For this review, take the finished solid that the model builds, in its own axes (mm). A direction names the side the tool comes from. Coordinates: 2 decimals unless noted, no trailing zeros. Write each loop counter-clockwise with the first axis right and the second up, starting at its lowest first coordinate (ties: lowest second). Pieces come first, ordered by that corner, then holes. Notation, with made-up numbers: M 53,13 L 79,13 A35 cw 79,48 Z; hole C 73.25,81.25 d11. An arc over 180 degrees is marked long. Return JSON: item names as keys, results as strings.
```python
from build123d import *

# Parameters (mm, degrees)
ESBO_O1_W                      = 4
ESBO_O1_H                      = 4
RESSALTO_EXTRUS_O1_DEPTH       = 100
PADR_OCIRCULAR1_COUNT          = 4
PADR_O_LINEAR1_COUNT           = 2
PADR_O_LINEAR1_PITCH           = 30
PADR_O_LINEAR1_COPY_1_SKETCH_W = 4
PADR_O_LINEAR1_COPY_1_SKETCH_H = 4
PADR_O_LINEAR1_COPY_1_DEPTH    = 100
PADR_O_LINEAR1_COPY_2_SKETCH_W = 4
PADR_O_LINEAR1_COPY_2_SKETCH_H = 4
PADR_O_LINEAR1_COPY_2_DEPTH    = 100
PADR_O_LINEAR1_COPY_3_SKETCH_W = 4
PADR_O_LINEAR1_COPY_3_SKETCH_H = 4
PADR_O_LINEAR1_COPY_3_DEPTH    = 100
ESBO_O4_W                      = 10
ESBO_O4_H                      = 28
CORTE_EXTRUS_O1_DEPTH          = 111.679718106
FILETE1_R                      = 1
CUT_EXTRUDE1_DEPTH             = 118.579760163


with BuildPart() as part:
    # Esboço1 → Ressalto-extrusão1 (new body)
    with BuildSketch(Plane.XY):
        with BuildLine():
            ThreePointArc((-1.664601464, 3.078815026), (-0.858529967, 3.393070335), (0, 3.5))
            Line((0, 3.5), (0, 6))
            Line((0, 6), (-3.878679656, 6))
            Line((-3.878679656, 6), (-8.5, 10.621320344))
            Line((-8.5, 10.621320344), (-8.5, 13))
            Line((-8.5, 13), (-4.1, 13))
            Line((-4.1, 13), (-4.1, 14.5))
            Line((-4.1, 14.5), (-5.1, 14.5))
            Line((-5.1, 14.5), (-5.1, 15))
            Line((-5.1, 15), (-15, 15))
            Line((-15, 15), (-15, 5.1))
            Line((-15, 5.1), (-14.5, 5.1))
            Line((-14.5, 5.1), (-14.5, 4.1))
            Line((-14.5, 4.1), (-13, 4.1))
            Line((-13, 4.1), (-13, 8.5))
            Line((-13, 8.5), (-10.621320344, 8.5))
            Line((-10.621320344, 8.5), (-6, 3.878679656))
            Line((-6, 3.878679656), (-6, 0))
            Line((-6, 0), (-3.5, 0))
            ThreePointArc((-3.5, 0), (-3.393070335, 0.858529967), (-3.078815026, 1.664601464))
            Line((-3.078815026, 1.664601464), (-4.596194078, 3.181980515))
            Line((-4.596194078, 3.181980515), (-3.181980515, 4.596194078))
            Line((-3.181980515, 4.596194078), (-1.664601464, 3.078815026))
        make_face()
        with Locations((-12, 12)):
            Rectangle(ESBO_O1_W, ESBO_O1_H, mode=Mode.SUBTRACT)
    ressalto_extrus_o1 = extrude(amount=RESSALTO_EXTRUS_O1_DEPTH)

    # PadrãoCircular1: Ressalto-extrusão1 ×4 about axis
    padr_ocircular1_axis = Axis((0, 0, 0), (0, 0, 1))
    for i in range(1, PADR_OCIRCULAR1_COUNT):
        add(ressalto_extrus_o1.rotate(padr_ocircular1_axis, i * 360 / PADR_OCIRCULAR1_COUNT))

    # Padrão linear1: Ressalto-extrusão1 ×2
    with Locations(*[(i * PADR_O_LINEAR1_PITCH, 0, 0) for i in range(1, PADR_O_LINEAR1_COUNT)]):
        add(ressalto_extrus_o1)

    # Padrão linear1 copy 1 sketch → Padrão linear1 copy 1 (add)
    with BuildSketch(Plane(origin=(30, 0, 0), x_dir=(0, 1, 0), z_dir=(0, 0, 1))):
        with BuildLine():
            ThreePointArc((-1.664601464, 3.078815026), (-0.858529967, 3.393070335), (0, 3.5))
            Line((0, 3.5), (0, 6))
            Line((0, 6), (-3.878679656, 6))
            Line((-3.878679656, 6), (-8.5, 10.621320344))
            Line((-8.5, 10.621320344), (-8.5, 13))
            Line((-8.5, 13), (-4.1, 13))
            Line((-4.1, 13), (-4.1, 14.5))
            Line((-4.1, 14.5), (-5.1, 14.5))
            Line((-5.1, 14.5), (-5.1, 15))
            Line((-5.1, 15), (-15, 15))
            Line((-15, 15), (-15, 5.1))
            Line((-15, 5.1), (-14.5, 5.1))
            Line((-14.5, 5.1), (-14.5, 4.1))
            Line((-14.5, 4.1), (-13, 4.1))
            Line((-13, 4.1), (-13, 8.5))
            Line((-13, 8.5), (-10.621320344, 8.5))
            Line((-10.621320344, 8.5), (-6, 3.878679656))
            Line((-6, 3.878679656), (-6, 0))
            Line((-6, 0), (-3.5, 0))
            ThreePointArc((-3.5, 0), (-3.393070335, 0.858529967), (-3.078815026, 1.664601464))
            Line((-3.078815026, 1.664601464), (-4.596194078, 3.181980515))
            Line((-4.596194078, 3.181980515), (-3.181980515, 4.596194078))
            Line((-3.181980515, 4.596194078), (-1.664601464, 3.078815026))
        make_face()
        with Locations((-12, 12)):
            Rectangle(PADR_O_LINEAR1_COPY_1_SKETCH_W, PADR_O_LINEAR1_COPY_1_SKETCH_H, mode=Mode.SUBTRACT)
    extrude(amount=PADR_O_LINEAR1_COPY_1_DEPTH)

    # Padrão linear1 copy 2 sketch → Padrão linear1 copy 2 (add)
    with BuildSketch(Plane(origin=(30, 0, 0), x_dir=(-1, 0, 0), z_dir=(0, 0, 1))):
        with BuildLine():
            ThreePointArc((-1.664601464, 3.078815026), (-0.858529967, 3.393070335), (0, 3.5))
            Line((0, 3.5), (0, 6))
            Line((0, 6), (-3.878679656, 6))
            Line((-3.878679656, 6), (-8.5, 10.621320344))
            Line((-8.5, 10.621320344), (-8.5, 13))
            Line((-8.5, 13), (-4.1, 13))
            Line((-4.1, 13), (-4.1, 14.5))
            Line((-4.1, 14.5), (-5.1, 14.5))
            Line((-5.1, 14.5), (-5.1, 15))
            Line((-5.1, 15), (-15, 15))
            Line((-15, 15), (-15, 5.1))
            Line((-15, 5.1), (-14.5, 5.1))
            Line((-14.5, 5.1), (-14.5, 4.1))
            Line((-14.5, 4.1), (-13, 4.1))
            Line((-13, 4.1), (-13, 8.5))
            Line((-13, 8.5), (-10.621320344, 8.5))
            Line((-10.621320344, 8.5), (-6, 3.878679656))
            Line((-6, 3.878679656), (-6, 0))
            Line((-6, 0), (-3.5, 0))
            ThreePointArc((-3.5, 0), (-3.393070335, 0.858529967), (-3.078815026, 1.664601464))
            Line((-3.078815026, 1.664601464), (-4.596194078, 3.181980515))
            Line((-4.596194078, 3.181980515), (-3.181980515, 4.596194078))
            Line((-3.181980515, 4.596194078), (-1.664601464, 3.078815026))
        make_face()
        with Locations((-12, 12)):
            Rectangle(PADR_O_LINEAR1_COPY_2_SKETCH_W, PADR_O_LINEAR1_COPY_2_SKETCH_H, mode=Mode.SUBTRACT)
    extrude(amount=PADR_O_LINEAR1_COPY_2_DEPTH)

    # Padrão linear1 copy 3 sketch → Padrão linear1 copy 3 (add)
    with BuildSketch(Plane(origin=(30, 0, 0), x_dir=(0, -1, 0), z_dir=(0, 0, 1))):
        with BuildLine():
            ThreePointArc((-1.664601464, 3.078815026), (-0.858529967, 3.393070335), (0, 3.5))
            Line((0, 3.5), (0, 6))
            Line((0, 6), (-3.878679656, 6))
            Line((-3.878679656, 6), (-8.5, 10.621320344))
            Line((-8.5, 10.621320344), (-8.5, 13))
            Line((-8.5, 13), (-4.1, 13))
            Line((-4.1, 13), (-4.1, 14.5))
            Line((-4.1, 14.5), (-5.1, 14.5))
            Line((-5.1, 14.5), (-5.1, 15))
            Line((-5.1, 15), (-15, 15))
            Line((-15, 15), (-15, 5.1))
            Line((-15, 5.1), (-14.5, 5.1))
            Line((-14.5, 5.1), (-14.5, 4.1))
            Line((-14.5, 4.1), (-13, 4.1))
            Line((-13, 4.1), (-13, 8.5))
            Line((-13, 8.5), (-10.621320344, 8.5))
            Line((-10.621320344, 8.5), (-6, 3.878679656))
            Line((-6, 3.878679656), (-6, 0))
            Line((-6, 0), (-3.5, 0))
            ThreePointArc((-3.5, 0), (-3.393070335, 0.858529967), (-3.078815026, 1.664601464))
            Line((-3.078815026, 1.664601464), (-4.596194078, 3.181980515))
            Line((-4.596194078, 3.181980515), (-3.181980515, 4.596194078))
            Line((-3.181980515, 4.596194078), (-1.664601464, 3.078815026))
        make_face()
        with Locations((-12, 12)):
            Rectangle(PADR_O_LINEAR1_COPY_3_SKETCH_W, PADR_O_LINEAR1_COPY_3_SKETCH_H, mode=Mode.SUBTRACT)
    extrude(amount=PADR_O_LINEAR1_COPY_3_DEPTH)

    # Esboço4 → Corte-extrusão1 (cut, through all)
    with BuildSketch(Plane(origin=(0, 0, 0), x_dir=(-1, 0, 0), z_dir=(0, 0, -1))):
        with Locations((-15, 0)):
            Rectangle(ESBO_O4_W, ESBO_O4_H)
    extrude(amount=-CORTE_EXTRUS_O1_DEPTH, mode=Mode.SUBTRACT)

    # Filete1
    filete1_edges = [part.edges().sort_by_distance(p)[0] for p in [
        (45, -15, 50),
        (45, 15, 50),
        (-15, 15, 50),
        (-15, -15, 50),
    ]]
    fillet(filete1_edges, radius=FILETE1_R)

    # Sketch1 → Cut-Extrude1 (cut, through all)
    with BuildSketch(Plane.ZY.offset(15)):
        Polygon((0, -15), (12.426406871, 15), (0, 15), align=None)
        Polygon((100, -15), (87.573593129, 15), (100, 15), align=None)
    extrude(amount=-CUT_EXTRUDE1_DEPTH, mode=Mode.SUBTRACT)


solid = part.part
```
1. For faces 4 (the face through (40, 15, 49)), 5 (the face through (0, 6, 49)), 6 (the face through (20, 11, 49)), list the 3-axis set-ups (+Z, -Z, +X, -X, +Y, -Y) from which the entire face can be reached by the end or side of a thin tool; tool diameter is ignored.
Checks:
{"face 4": "+Z, -Z, +X, -X, +Y", "face 5": "+Z, -Z, +Y", "face 6": "+Z, -Z"}
2. Draft analysis for pull direction X (two halves, no side actions). For faces 1 (the face through (-6, 0, 49)), 2 (the face through (36, 0, 49)), 3 (the face through (8.5, -12, 49)), state which applies: +X half, -X half, draft (parallel to the pull), parting line (faces both ways), or undercut.
Checks:
{"face 1": "-X half", "face 2": "+X half", "face 3": "undercut"}
3. We need section B-B (z = 25). Give the number of separate pieces and of enclosed holes in the cut face, plus the area to 3 significant figures.
Checks:
{"separate pieces": "1", "enclosed holes": "7", "area": "561 mm2"}
4. Wall thickness on L1, parallel to X at y = 13.25, z = 53; L2, parallel to X at y = 0.25, z = 31; L3, parallel to X at y = 1.5, z = 91: over which ranges is each line inside the solid? List them lowest first. Write a range as from..to.
Checks:
{"L1": "-15..-14, -10..-4.1, 4.1..10, 20..25.9, 34.1..40, 44..45", "L2": "-6..-3.49, 3.49..6, 24..26.51, 33.49..36", "L3": "-6..-3.16, 3.16..6, 24..26.84, 33.16..36"}
5. We need section A-A (y = -11.75). State the section outline as (x, z) points, plus the area to 3 significant figures.
Checks:
{"outline": "M -15,1.35 L -14,1.35 L -14,98.65 L -15,98.65 Z; M -10,1.35 L -8.5,1.35 L -8.5,98.65 L -10,98.65 Z; M 8.5,1.35 L 10,1.35 L 10,98.65 L 8.5,98.65 Z; M 20,1.35 L 21.5,1.35 L 21.5,98.65 L 20,98.65 Z; M 38.5,1.35 L 40,1.35 L 40,98.65 L 38.5,98.65 Z; M 44,1.35 L 45,1.35 L 45,98.65 L 44,98.65 Z", "area": "778 mm2"}
6. Clearance check with flat-ended pins moving along their axes: pin 1 Ø8 at (x, z) = (32, 30.5) entering from +Y; pin 2 Ø0.8 at (x, z) = (34.5, 64.5) entering from +Y; pin 3 Ø2.5 at (y, z) = (1.5, 52) entering from +X; pin 4 Ø8 at (x, y) = (18.5, 1.5) entering from -Z. State where each tip first meets the part, or that it passes through.
Checks:
{"pin 1": "y = 15", "pin 2": "y = 14.5", "pin 3": "x = 36", "pin 4": "through"}
